Work out the finished part from the listing and answer in its coordinate system (mm). Face numbers are marked on the shaded views. A direction names the side the tool comes from. Coordinates: 2 decimals unless noted, no trailing zeros. Order: outer loops, then holes, each group sorted by start corner. A loop starts at its lowest first (then second) coordinate and runs counter-clockwise, first axis right, second up.
```python
from build123d import *

# Parameters (mm, degrees)
CHANFREIN1_SIZE         = 0.2
CONG_1_R                = 0.2
ENL_V_MAT_EXTRU_1_DEPTH = 1.3


with BuildPart() as part:
    # Esquisse1 → Révolution1 (revolve)
    with BuildSketch(Plane.XY):
        Polygon((0, 0), (0, 2.75), (3, 2.75), (3, 1.5), (11, 1.5), (11, 0), align=None)
    revolve(axis=Axis((0, 0, 0), (1, 0, 0)))

    # Chanfrein1
    chanfrein1_edges = [part.edges().sort_by_distance(p)[0] for p in [
        (11, -1.5, 0),
    ]]
    chamfer(chanfrein1_edges, length=CHANFREIN1_SIZE)

    # Congé1
    cong_1_edges = [part.edges().sort_by_distance(p)[0] for p in [
        (3, -1.5, 0),
        (0, -2.75, 0),
    ]]
    fillet(cong_1_edges, radius=CONG_1_R)

    # Esquisse2 → Enlèv. mat.-Extru.1 (cut)
    with BuildSketch(Plane.ZY):
        Polygon((0.739008345, -1.28), (1.478016689, 0), (0.739008345, 1.28), (-0.739008345, 1.28), (-1.478016689, 0), (-0.739008345, -1.28), align=None)
    extrude(amount=-ENL_V_MAT_EXTRU_1_DEPTH, mode=Mode.SUBTRACT)


solid = part.part
```
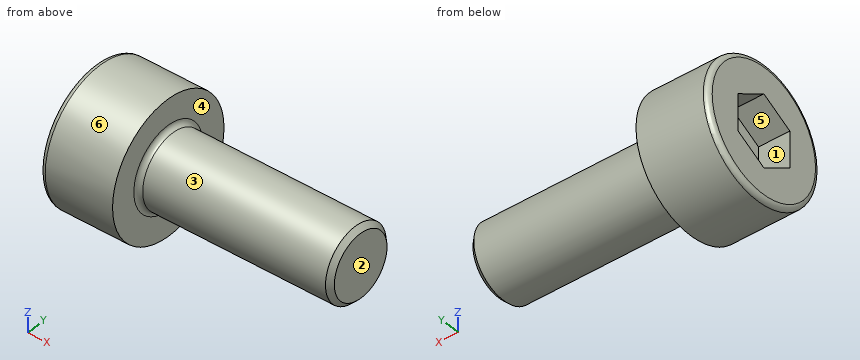
1. The part is cut by section B-B (z = 0). Determine the outline of the cut face in (x, y), plus the area to 3 significant figures.
2. The part is cut by section C-C (x = 3.5). Determine the outline of the cut face in (y, z).
3. Consider probe 1 along X at (y, z) = (-0.2, -0.6); probe 2 along X at (y, z) = (-2.2, -1.25); probe 3 along Z at (x, y) = (7.5, 0.1). Determine where each line is inside the solid, lowest interval first.
4. The mould has two halves that part along Z. Classify the marked faces 1, 2 and 3: released by +Z, released by -Z, zero draft, split by the parting line, or undercut.
5. The part is cut by section A-A (x = 0.5). Determine the outline of the cut face in (y, z), plus the area to 3 significant figures.
6. For the marked faces 4, 5 and 6, determine the directions among +Z, -Z, +X, -X, +Y, -Y from which every point of the face is accessible in a straight line to the end or side of a thin tool.
Worked out:
1. outline: (0, -2.55) arc R0.2 ccw to (0.2, -2.75) - (3, -2.75) - (3, -1.7) arc R0.2 cw to (3.2, -1.5) - (10.8, -1.5) - (11, -1.3) - (11, 1.3) - (10.8, 1.5) - (3.2, 1.5) arc R0.2 cw to (3, 1.7) - (3, 2.75) - (0.2, 2.75) arc R0.2 ccw to (0, 2.55) - (0, 1.28) - (1.3, 1.28) - (1.3, -1.28) - (0, -1.28) - close
1. area: 37.1 mm2
2. outline: circle Ø3 at (0, 0)
3. probe 1: x = 1.3 to 11
3. probe 2: x = 0 to 3
3. probe 3: z = -1.5 to 1.5
4. face 1: undercut
4. face 2: zero draft
4. face 3: split by the parting line
5. outline: circle Ø5.5 at (0, 0); hole (-1.28, -0.74) - (0, -1.48) - (1.28, -0.74) - (1.28, 0.74) - (0, 1.48) - (-1.28, 0.74) - close
5. area: 18.1 mm2
6. face 4: +X
6. face 5: -X
6. face 6: +X, -X
